Build history of the part. All positions in model axes, mm. Face numbers are marked on the shaded views. A direction names the side the tool comes from. Give positions to 0.01 mm unless a question says otherwise; leave off trailing zeros. Order: outer loops, then holes, each group sorted by start corner. A loop starts at its lowest first (then second) coordinate and runs counter-clockwise, first axis right, second up. Notation, with made-up numbers: (19, 34.5) - (24, 34.5) arc R28 cw to (24, 71.5) - close; hole circle Ø10 at (10.25, 10.25). An arc over 180 degrees is marked (long way). Use a Markdown table: item, result.
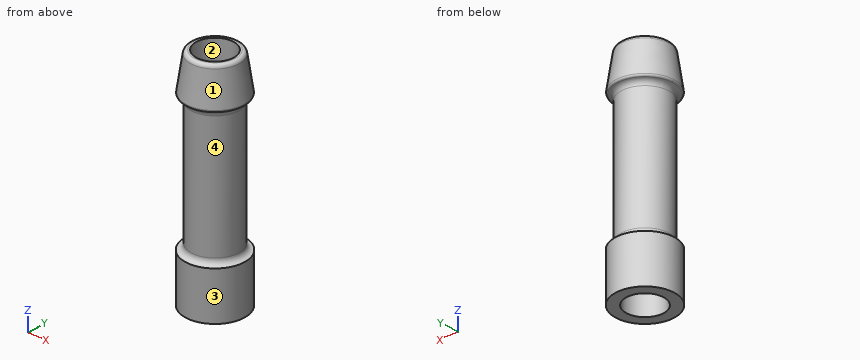
from build123d import *

# Parameters (mm, degrees)
SKETCH1_R           = 3.937
BOSS_EXTRUDE1_DEPTH = 29.21
SKETCH2_R           = 2.5
CUT_EXTRUDE1_START  = -5.08
SKETCH3_R           = 5.08
SKETCH3_R_2         = 3.175
CUT_EXTRUDE1_DEPTH  = 17.78
FILLET1_R           = 0.762
FILLET2_R           = 0.762
CHAMFER1_SIZE       = 5.08
CHAMFER1_SIZE_2     = 0.759211087
FILLET3_R           = 0.254
FILLET4_R           = 0.508


# Some blends are built 0.0001 mm under size
with BuildPart() as part:
    # Sketch1 → Boss-Extrude1 (new body)
    with BuildSketch(Plane.XY):
        with Locations(Location((0, 0, 0), (0, 0, 180))):
            Circle(SKETCH1_R)
    extrude(amount=BOSS_EXTRUDE1_DEPTH)

    # Cut-Sweep1: sweep along a curve in space
    with BuildLine() as cut_sweep1_path:
        Line((0, 0, 29.21), (0, 0, 0))
    # Sketch2 → Cut-Sweep1 (sweep, cut)
    with BuildSketch(Plane.XY.offset(29.21)):
        Circle(SKETCH2_R)
    sweep(path=cut_sweep1_path.line, mode=Mode.SUBTRACT)

    # Sketch3 → Cut-Extrude1 (cut)
    with BuildSketch(Plane.XY.offset(29.21).offset(CUT_EXTRUDE1_START)):
        Circle(SKETCH3_R)
        Circle(SKETCH3_R_2, mode=Mode.SUBTRACT)
    extrude(amount=-CUT_EXTRUDE1_DEPTH, mode=Mode.SUBTRACT)

    # Fillet1
    fillet1_edges = [part.edges().sort_by_distance(p)[0] for p in [
        (-3.175, 0, 6.35),
    ]]
    fillet(fillet1_edges, radius=FILLET1_R - 0.0001)  # a hair under: the kernel refuses the full size

    # Fillet2
    fillet2_edges = [part.edges().sort_by_distance(p)[0] for p in [
        (-3.175, 0, 24.13),
    ]]
    fillet(fillet2_edges, radius=FILLET2_R - 0.0001)  # a hair under: the kernel refuses the full size

    # Chamfer1
    # the kernel refuses this chamfer: 5.08, 0.759211087 mm, written as the material it takes off along each edge
    with BuildSketch(Plane(origin=(0, 0, 29.21), x_dir=(-1, 0, 0), z_dir=(0, 1, 0))) as chamfer1_piece_1:
        Polygon((3.937, -CHAMFER1_SIZE), (3.937 - CHAMFER1_SIZE_2, 0), (3.937, 0), align=None)
    revolve(axis=Axis((0, 0, 29.21), (0, 0, 1)), mode=Mode.SUBTRACT)

    # Fillet3
    fillet3_edges = [part.edges().sort_by_distance(p)[0] for p in [
        (3.937, 0, 24.13),
    ]]
    fillet(fillet3_edges, radius=FILLET3_R)

    # Fillet4
    fillet4_edges = [part.edges().sort_by_distance(p)[0] for p in [
        (3.177788913, 0, 29.21),
    ]]
    fillet(fillet4_edges, radius=FILLET4_R)


solid = part.part
1) Pin check, flat tip, straight feed: P1, Ø4, axis at y = 0, z = 18, coming from the -X side (3 decimals). Stop position of the tip, or through.
Computed:
| item | result |
|---|---|
| P1 | stops at x = -3.175 |
2) Two-plate mould, pull along Y, no slides. Class the marked faces 1 and 2: +Y half, -Y half, draft (parallel to the pull), parting line (faces both ways), or undercut.
Computed:
| item | result |
|---|---|
| face 1 | parting line |
| face 2 | undercut |
3) Wall check: line 1 (Y direction, x = 0, z = 22.5) (3 decimals); line 2 (X direction, y = 1, z = 8); line 3 (Y direction, x = 1.75, z = 7.5). Give the ranges that are in metal, low to high. Write a range as from..to.
Computed:
| item | result |
|---|---|
| line 1 | y = -3.175..-2.5, 2.5..3.175 |
| line 2 | x = -3.01..-2.29, 2.29..3.01 |
| line 3 | y = -2.65..-1.79, 1.79..2.65 |
4) Slice it at A-A (z = 4.25). Write the cut outline in (x, y), and give its area (3 significant figures).
Computed:
| item | result |
|---|---|
| outline | circle Ø7.87 at (0, 0); hole circle Ø5 at (0, 0) |
| area | 29.1 mm² |
5) Tool access for the marked faces 3 and 4: list every direction of +Z, -Z, +X, -X, +Y, -Y with a clear straight run to the whole face (end or side of a thin tool).
Computed:
| item | result |
|---|---|
| face 3 | +Z, -Z |
| face 4 | none |
6) Slice it at B-B (z = 16). Write the cut outline in (x, y) (3 decimals), and give its area (3 significant figures).
Computed:
| item | result |
|---|---|
| outline | circle Ø6.35 at (0, 0); hole circle Ø5 at (0, 0) |
| area | 12.0 mm² |
